The model under review builds one solid part; all positions refer to its coordinate system, in mm. A direction names the side the tool comes from. Give positions to 0.01 mm unless a question says otherwise; leave off trailing zeros. Order: outer loops, then holes, each group sorted by start corner. A loop starts at its lowest first (then second) coordinate and runs counter-clockwise, first axis right, second up. Notation, with made-up numbers: (89.25, -37) - (125.25, -37) arc R16 ccw to (125.25, -29) - close; hole circle Ø6 at (82, -36). An arc over 180 degrees is marked (long way). Use a Markdown table: item, result. Add a question column.
```python
from build123d import *

# Parameters (mm, degrees)
F0_W     = 825
F0_H     = 100
F1_DEPTH = 200
F2_T     = -1
F5_D     = 20
F8_D     = 30


# Not quite as in the source:
# - the program builds the solid bodies; features that only make, move or delete a surface that nothing else refers to are left out


with BuildPart() as f1:
    # F0 (on Top) → F1 (new body)
    with BuildSketch(Plane.XY):
        Rectangle(F0_W, F0_H)
    extrude(amount=F1_DEPTH)

    # F2
    f2_openings = [f1.faces().sort_by_distance(p)[0] for p in [
        (0, 0, 200),
    ]]
    offset(amount=F2_T, openings=f2_openings)

    # F5 (through all)
    with Locations(Plane.XY.offset(1)):
        with Locations((399.5, 37), (399.5, -37), (-399.5, 37), (-399.5, -37)):
            Hole(F5_D / 2)

    # F8 (through all)
    with Locations(Plane(origin=(-412.5, 0, 0), x_dir=(0, -1, 0), z_dir=(-1, 0, 0))):
        with Locations((0, 50)):
            Hole(F8_D / 2)


solid = f1.part
```
Q1. We need section B-B (x = -399.5). Write out the cut boundary in (y, z), plus the area to 3 significant figures.
Q2. We need section A-A (y = -37). Write out the cut boundary in (x, z).
Q3. Clearance check with flat-ended pins moving along their axes: P1, Ø3, axis at x = -187.5, y = -25, coming from the +Z side; P2, Ø12, axis at x = -399.5, y = -37, coming from the -Z side. State where each tip first meets the part, or that it passes through.
Q4. Draft analysis for pull direction Y (two halves, no side actions). For faces 3 (the cylindrical face through (-411.993, -1.953, 64.872)), 4 (the flat face through (-6, -50, 99)), 5 (the flat face through (-6, 50, 99)), 6 (the flat face through (411.5, -1, 99)), state which applies: pulls with the +Y half, pulls with the -Y half, needs draft (parallel to the pull), parting line crosses it, or undercut.
Q5. We need section C-C (z = 132). Write out the cut boundary in (x, y), plus the area to 3 significant figures.
Q6. Wall thickness on probe 1 along Y at (x, z) = (-362.5, 176.5); probe 2 along Y at (x, z) = (-399.5, 0.7); probe 3 along X at (y, z) = (-23, 40.5): over which ranges is each line inside the solid? List them lowest first.
Q7. We need section D-D (z = 50). Write out the cut boundary in (x, y), plus the area to 3 significant figures.
Q8. Machinability: for faces 1 (the flat face through (-412.5, -1, 99)), 2 (the flat face through (-411.5, -1, 99)), which of the approach directions +Z, -Z, +X, -X, +Y, -Y give a long, thin tool a straight path to every point of the face, cutting with its end or side? Answer none if there is none.
Here are the results:
| question | item | result |
|---|---|---|
| 1 | outline | (-50, 0) - (-47, 0) - (-47, 1) - (-49, 1) - (-49, 200) - (-50, 200) - close; (-27, 0) - (27, 0) - (27, 1) - (-27, 1) - close; (47, 0) - (50, 0) - (50, 200) - (49, 200) - (49, 1) - (47, 1) - close |
| 1 | area | 458 mm2 |
| 2 | outline | (-412.5, 0) - (-409.5, 0) - (-409.5, 1) - (-411.5, 1) - (-411.5, 200) - (-412.5, 200) - close; (-389.5, 0) - (389.5, 0) - (389.5, 1) - (-389.5, 1) - close; (409.5, 0) - (412.5, 0) - (412.5, 200) - (411.5, 200) - (411.5, 1) - (409.5, 1) - close |
| 3 | P1 | z = 1 |
| 3 | P2 | through |
| 4 | face 3 | undercut |
| 4 | face 4 | pulls with the -Y half |
| 4 | face 5 | pulls with the +Y half |
| 4 | face 6 | undercut |
| 5 | outline | (-412.5, -50) - (412.5, -50) - (412.5, 50) - (-412.5, 50) - close; hole (-411.5, -49) - (411.5, -49) - (411.5, 49) - (-411.5, 49) - close |
| 5 | area | 1,850 mm2 |
| 6 | probe 1 | -50 to -49, 49 to 50 |
| 6 | probe 2 | -50 to -47, -27 to 27, 47 to 50 |
| 6 | probe 3 | -412.5 to -411.5, 411.5 to 412.5 |
| 7 | outline | (-412.5, -50) - (412.5, -50) - (412.5, -15) - (411.5, -15) - (411.5, -49) - (-411.5, -49) - (-411.5, -15) - (-412.5, -15) - close; (-412.5, 15) - (-411.5, 15) - (-411.5, 49) - (411.5, 49) - (411.5, 15) - (412.5, 15) - (412.5, 50) - (-412.5, 50) - close |
| 7 | area | 1,790 mm2 |
| 8 | face 1 | +Z, -Z, -X, +Y, -Y |
| 8 | face 2 | +Z |
